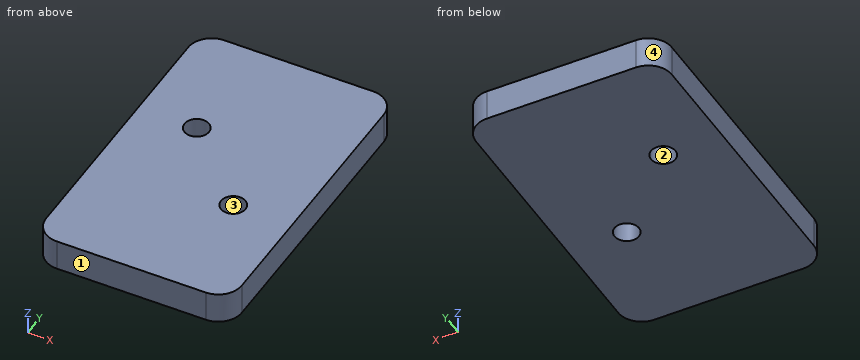
```python
from build123d import *

# Parameters (mm, degrees)
SKETCH_W  = 25
SKETCH_H  = 40
SKETCH_R  = 1.5625
PAD_DEPTH = 4
FILLET_R  = 3


with BuildPart() as part:
    # Sketch → Pad (new body)
    with BuildSketch(Plane.XY):
        with Locations((25, 20)):
            Rectangle(SKETCH_W, SKETCH_H)
        with Locations((20, 25)):
            Circle(SKETCH_R, mode=Mode.SUBTRACT)
        with Locations((30, 15)):
            Circle(SKETCH_R, mode=Mode.SUBTRACT)
    extrude(amount=PAD_DEPTH)

    # Fillet
    fillet_edges = [part.edges().sort_by_distance(p)[0] for p in [
        (12.5, 0, 2),
        (12.5, 40, 2),
        (37.5, 40, 2),
        (37.5, 0, 2),
    ]]
    fillet(fillet_edges, radius=FILLET_R)


solid = part.part
```
Part model, mm, in its own coordinate system. Face numbers are marked on the shaded views. Coordinates: 2 decimals unless noted, no trailing zeros. Loops run counter-clockwise (first coordinate to the right, second up) from the corner with the lowest first, then second, coordinate; pieces in that order, holes last. Notation, with made-up numbers: (16.25, -38) - (26.25, -38) arc R19 ccw to (26.25, -9) - close; hole circle Ø10 at (-10.75, 77). An arc over 180 degrees is marked (long way). Write item = value, one per line. Start each with the question number.
Item 1: Mould opens along X. For the marked faces 1, 2, 3 and 4 say: released by +X, released by -X, zero draft, split by the parting line, or undercut.
Item 2: Wall check: L1, parallel to Y at x = 30, z = 1.5; L2, parallel to Y at x = 20, z = 1.7; L3, parallel to X at y = 14, z = 0.5. Give the ranges that are in metal, low to high. Write a range as from..to.
Item 3: Cut at B-B, the plane x = 20. Give the cut face in (y, z), and give its area (4 significant figures).
Item 4: Flat gauge pin, fed straight in: pin 1 Ø1.9 at (x, y) = (20, 25) entering from +Z. Where does the tip first touch, or does it go through?
Item 5: Cut at C-C, the plane z = 1. Give the cut face in (x, y) (1 decimal).
Item 6: Cut at A-A, the plane y = 25. Give the cut face in (x, z).
The answers:
q1.face_1 = zero draft
q1.face_2 = undercut
q1.face_3 = undercut
q1.face_4 = released by -X
q2.L1 = 0..13.44, 16.56..40
q2.L2 = 0..23.44, 26.56..40
q2.L3 = 12.5..28.8, 31.2..37.5
q3.outline = (0, 0) - (23.44, 0) - (23.44, 4) - (0, 4) - close; (26.56, 0) - (40, 0) - (40, 4) - (26.56, 4) - close
q3.area = 147.5 mm2
q4.pin_1 = through
q5.outline = (12.5, 3) arc R3 ccw to (15.5, 0) - (34.5, 0) arc R3 ccw to (37.5, 3) - (37.5, 37) arc R3 ccw to (34.5, 40) - (15.5, 40) arc R3 ccw to (12.5, 37) - close; hole circle Ø3.1 at (20, 25); hole circle Ø3.1 at (30, 15)
q6.outline = (12.5, 0) - (18.44, 0) - (18.44, 4) - (12.5, 4) - close; (21.56, 0) - (37.5, 0) - (37.5, 4) - (21.56, 4) - close
